Check sheet for the modelled part. Datum: model origin and axes. Units: mm. A direction names the side the tool comes from. Give positions to 0.01 mm unless a question says otherwise; leave off trailing zeros. Loops run counter-clockwise (first coordinate to the right, second up) from the corner with the lowest first, then second, coordinate; pieces in that order, holes last. Notation, with made-up numbers: (42.5, 82.5) -> (70.5, 82.5) arc R25 ccw to (70.5, 104.5) -> close; hole circle Ø4 at (88.5, 75). An arc over 180 degrees is marked (long way). Answer as CSV lines item,"result". Start each with the question number.
(1) Gauge pin test, flat ends, axial feed: pin 1 Ø5.5 at (y, z) = (19.05, 9.18) entering from -X; pin 2 Ø10.5 at (y, z) = (17, 9) entering from +X; pin 3 Ø5 at (y, z) = (44.5, 5.5) entering from -X. Record the tip position at first contact, or that the pin passes through.
(2) Section check B-B on y = 64.5. Enter the section's corners in (x, z), plus the area to 3 significant figures.
(3) Material ranges on line 1 (Y direction, x = 17.5, z = 31.5); line 2 (Y direction, x = 24.5, z = -2.5); line 3 (X direction, y = 68, z = -1), recorded low to high. Write a range as from..to.
(4) Release check for a two-part mould opening along X. For faces 1 (the face through (-7.938, 59, 7)), 2 (the face through (7.938, 21, 7)), 3 (the face through (-15.12, 18.96, -11.59)), 4 (the face through (6.391, 75.395, 3.767)) record: pulls with the +X half, pulls with the -X half, needs draft (parallel to the pull), parting line crosses it, or undercut.
(5) Section check A-A on x = 0. State how many separate pieces and enclosed holes the cut face has, plus the area to 3 significant figures.
(6) Access from +Z, -Z, +X, -X, +Y, -Y to the whole of each face (thin tool, end or side, straight path). Record for faces 5 (the face through (10.241, 57.237, -16.063)), 6 (the face through (-6.391, 75.395, -3.767)), 7 (the face through (-6.41, 0.78, 3.78)), 8 (the face through (5.774, 37.589, -3.271)).
Autodesk Inventor part; units mm, degrees
ref_plane "Work Plane4" through (-19.05, 0, 0) normal (1, 0, 0) x (0, 1, 0)
ref_plane "Work Plane5" through (19.05, 0, 0) normal (1, 0, 0) x (0, 1, 0)
ref_plane "XZ Plane" through (0, 0, 0) normal (0, 1, 0) x (-1, 0, 0)
sketch "Sketch15" plane through (0, 0, 0) normal (0, 0, 1) x (1, 0, 0)
  line L0 (41.275, 0) -> (41.275, 76.2) construction
  line L1 (0, 0) -> (41.275, 0)
  line L2 (0, 76.2) -> (41.275, 76.2)
  line L3 (19.05, 0) -> (19.05, 76.2) construction
  line L4 (0, 76.2) -> (0, 0)
  line L5 (19.05, 19.05) -> (41.275, 19.05) construction
  line L6 (41.275, 0) -> (19.05, 12.8316)
  line L7 (41.275, 38.1) -> (19.05, 25.2684)
  line L8 (19.05, 25.2684) -> (41.275, 25.2684) construction
  line L9 (19.05, 25.2684) -> (19.05, 12.8316)
  line L10 (41.275, 38.1) -> (19.05, 50.9316)
  line L11 (19.05, 50.9316) -> (19.05, 63.3684)
  line L12 (19.05, 63.3684) -> (41.275, 76.2)
  line L13 (41.275, 38.1) -> (19.05, 38.1) construction
  line L14 (19.05, 63.3684) -> (41.275, 63.3684) construction
  dimension "d85" = 41.275
  dimension "d86" = 76.2
  dimension "d87" = 19.05
  dimension "d88" = 41.275
  dimension "d89" = 38.1
  dimension "centerLineForSpool" = 19.05
  dimension "d93" = 30
  dimension "d94" = 30
  dimension "d95" = 30
  dimension "d96" = 30
revolve "Revolution2" add sketch "Sketch15" angle 360 about axis through (0, 76.2, 0) along (0, -1, 0)
sketch "Sketch16" plane through (0, 0, 0) normal (0, -1, 0) x (1, 0, 0)
  line L0 (-7.6623, 0) -> (-3.8312, 6.6357)
  line L1 (-3.8312, 6.6357) -> (3.8312, 6.6357)
  line L2 (3.8312, 6.6357) -> (7.6623, 0)
  line L3 (7.6623, 0) -> (3.8312, -6.6358)
  line L4 (3.8312, -6.6358) -> (-3.8312, -6.6358)
  line L5 (-3.8312, -6.6358) -> (-7.6623, 0)
  point P0 (0, 0)
  point P1 (0, 0)
  dimension "d103" = 13.2715
extrude "Extrusion11" cut sketch "Sketch16" against normal through all
sketch "Sketch17" plane through (0, 0, 0) normal (1, 0, 0) x (0, 1, 0)
  circle A0 centre (57.15, 9.1757) radius 2.54
  circle A1 centre (19.05, 9.1757) radius 2.54
  line L0 (0, 41.275) -> (0, -41.275)
  line L1 (76.2, 41.275) -> (76.2, -41.275)
  line L2 (0, 6.6357) -> (76.2, 6.6357)
  point P0 (0, 0)
  dimension "d110" = 19.05
  dimension "d111" = 19.05
  dimension "d112" = 5.08
extrude "Extrusion13" cut sketch "Sketch17" along normal through all both and the other way through all
ref_plane "Work Plane4" through (-19.05, 0, 0) normal (1, 0, 0) x (0, 1, 0)
sketch "Sketch22" plane through (-19.05, 0, 0) normal (1, 0, 0) x (0, 1, 0)
  spline S0 degree 8 poles (59.69, 9.1757) (59.69, 9.4517) (59.6557, 9.7212) (59.59, 9.9804) (59.4956, 10.2261) (59.3755, 10.4557) (59.2323, 10.6669) (59.0691, 10.858) (58.7144, 11.191) (58.5225, 11.336) (58.3154, 11.4599) (58.0958, 11.5609) (57.8667, 11.6378) (57.6308, 11.6896) (57.3909, 11.7157) (56.8686, 11.7157) (56.5893, 11.6801) (56.3163, 11.6098) (56.0539, 11.5059) (55.8062, 11.37) (55.5775, 11.2041) (55.3719, 11.0111) (55.0147, 10.5794) (54.8595, 10.3366) (54.7333, 10.0693) (54.6415, 9.7817) (54.5882, 9.479) (54.5771, 9.1672) (54.6105, 8.8531) (54.8032, 8.1024) (55.0034, 7.6991) (55.2751, 7.3483) (55.6037, 7.0608) (55.9729, 6.8444) (56.3656, 6.703) (56.7635, 6.6357) (57.4276, 6.6357) (57.7065, 6.6704) (57.9827, 6.7403) (58.2517, 6.8459) (58.509, 6.9871) (58.7494, 7.1637) (58.9676, 7.3748) (59.2832, 7.7816) (59.3962, 7.9584) (59.4932, 8.1474) (59.5721, 8.3459) (59.6315, 8.5511) (59.6708, 8.76) (59.69, 8.9692) (59.69, 9.1757) knots 0 0 0 0 0 0 0 0 0 0.129052 0.129052 0.129052 0.129052 0.129052 0.129052 0.129052 0.253777 0.253777 0.253777 0.253777 0.253777 0.253777 0.253777 0.399469 0.399469 0.399469 0.399469 0.399469 0.399469 0.399469 0.544533 0.544533 0.544533 0.544533 0.544533 0.544533 0.544533 0.751894 0.751894 0.751894 0.751894 0.751894 0.751894 0.751894 0.900801 0.900801 0.900801 0.900801 0.900801 0.900801 0.900801 1 1 1 1 1 1 1 1 1
  circle A0 centre (57.15, 9.1757) radius 4.7625
  circle A1 centre (57.15, 9.1757) radius 2.54 construction
  line L0 (57.15, 6.6357) -> (76.2, 6.6357) construction
  line L1 (76.2, 41.275) -> (76.2, -41.275) construction
  point P0 (0, 0)
  dimension "d121" = 19.05
  dimension "d122" = 5.08
  dimension "d125" = 9.525
extrude "Extrusion16" cut sketch "Sketch22" along normal blind 11.1125
ref_plane "Work Plane5" through (19.05, 0, 0) normal (1, 0, 0) x (0, 1, 0)
sketch "Sketch23" plane through (19.05, 0, 0) normal (1, 0, 0) x (0, 1, 0)
  line L0 (19.05, 6.6357) -> (57.15, 6.6357)
  circle A0 centre (19.05, 9.1757) radius 2.54 construction
  line L1 (0, 41.275) -> (0, -41.275)
  circle A1 centre (19.05, 9.1757) radius 4.7625
  point P0 (0, 0)
  dimension "d127" = 5.08
  dimension "d128" = 19.05
  dimension "d129" = 9.525
extrude "Extrusion17" cut sketch "Sketch23" against normal blind 11.1125
chamfer "Chamfer10" distance 1.5875 angle 45 12 edges at (0, 76.2, -6.6358) (5.7467, 76.2, -3.3179) (5.7467, 76.2, 3.3179) (0, 76.2, 6.6357) (-5.7467, 76.2, 3.3179) (-5.7467, 76.2, -3.3179) (-5.7467, 0, -3.3179) (-5.7467, 0, 3.3179) (0, 0, 6.6357) (5.7467, 0, 3.3179) (5.7467, 0, -3.3179) (0, 0, -6.6358)
equation "\"d85\" = spoolExteriorRadius"
equation "\"d86\" = spoolOverallHeight"
equation "\"d88\" = d85"
equation "\"d89\" = 0.5 * spoolOverallHeight"
equation "\"centerLineForSpool\" = 0.25 * spoolOverallHeight"
equation "\"d103\" = hexDiameter"
equation "\"d110\" = centerLineForSpool"
equation "\"d111\" = centerLineForSpool"
equation "\"d112\" = holeForString"
equation "\"d121\" = centerLineForSpool"
equation "\"d122\" = holeForString"
equation "\"d125\" = knotHoleDiameter"
equation "\"d127\" = holeForString"
equation "\"d128\" = centerLineForSpool"
equation "\"d129\" = knotHoleDiameter"
equation "\"d130\" = knotHoleDepth"
equation "\"d132\" = hexHoleChamfer"
equation "\"holeForString\" = stringDiameter + clearanceForString"
equation "\"stringDiameter\" = 3.048"
equation "\"clearanceForString\" = 2.032"
equation "\"spoolHeightWithoutSpacer\" = 69.85"
equation "\"hexShaftDiameter\" = 12.7"
equation "\"clearanceForHexShaft\" = 0.5715"
equation "\"hexDiameter\" = hexShaftDiameter + clearanceForHexShaft"
equation "\"supportChannels\" = 3.81"
equation "\"spoolInteriorDiameter\" = 38.1"
equation "\"spoolInteriroRadius\" = 0.5 * spoolInteriorDiameter"
equation "\"spoolExteriorDiameter\" = 82.55"
equation "\"spoolExteriorRadius\" = 0.5 * spoolExteriorDiameter"
equation "\"spoolFiletRadius\" = 0.5 * supportChannels"
equation "\"holeCenter\" = 0.25 * spoolHeightWithoutSpacer - 0.75 * supportChannels"
equation "\"hexHoleChamfer\" = 1.5875"
equation "\"stringHoleCenterFromHexShaft\" = 0.5 * hexDiameter + 0.5 * holeForString"
equation "\"textCircleDiameter\" = 0.75 * spoolExteriorDiameter"
equation "\"textHeight\" = 6.096"
equation "\"textDepth\" = 1.27"
equation "\"stringHoleChamfer\" = 4.7625"
equation "\"spoolTotalHeight\" = 76.2"
equation "\"spaceHeight\" = spoolTotalHeight - spoolHeightWithoutSpacer"
equation "\"spacerDiameter\" = 24.13"
equation "\"spoolOverallHeight\" = 76.2"
equation "\"d114\" = -spoolInteriroRadius"
equation "\"knotHoleDiameter\" = 9.525"
equation "\"d126\" = spoolInteriroRadius"
properties part number "spoolV06" material "PC/ABS Plastic"
Working result:
1,pin 1,"stops at x = -17.93"
1,pin 2,"stops at x = 19.16"
1,pin 3,"stops at x = -34.1"
2,outline,"circle Ø42.02 at (0, 0); hole (-7.66, 0) -> (-3.83, -6.64) -> (3.83, -6.64) -> (7.66, 0) -> (3.83, 6.64) -> (-3.83, 6.64) -> close"
2,area,"1,230 mm^2"
3,line 1,"y = 0..3.03, 35.07..41.13, 73.17..76.2"
3,line 2,"y = 0..9.61, 28.49..47.71, 66.59..76.2"
3,line 3,"x = -27.05..-7.08, 7.08..27.05"
4,face 1,"pulls with the -X half"
4,face 2,"pulls with the +X half"
4,face 3,"parting line crosses it"
4,face 4,"undercut"
5,separate pieces,"2"
5,enclosed holes,"2"
5,area,"2,990 mm^2"
6,face 5,"none"
6,face 6,"+Y"
6,face 7,"-Y"
6,face 8,"+Y, -Y"
